```python
from build123d import *

# Parameters (mm, degrees)
SKETCH1_W           = 198.12
SKETCH1_H           = 248.92
SKETCH1_R           = 2.5
BOSS_EXTRUDE1_DEPTH = 3.175
SKETCH2_R           = 6.35
CUT_EXTRUDE1_DEPTH  = 4.175


with BuildPart() as part:
    # Sketch1 → Boss-Extrude1 (new body)
    with BuildSketch(Plane.XY):
        with Locations((0, -152.4)):
            Rectangle(SKETCH1_W, SKETCH1_H)
        with Locations((-76.2, -260.35)):
            Circle(SKETCH1_R, mode=Mode.SUBTRACT)
        with Locations((-76.2, -38.1)):
            Circle(SKETCH1_R, mode=Mode.SUBTRACT)
        with Locations((76.2, -38.1)):
            Circle(SKETCH1_R, mode=Mode.SUBTRACT)
        with Locations((76.2, -260.35)):
            Circle(SKETCH1_R, mode=Mode.SUBTRACT)
    extrude(amount=BOSS_EXTRUDE1_DEPTH)

    # Sketch2 → Cut-Extrude1 (cut, through all)
    with BuildSketch(Plane.XY.offset(3.175)):
        with Locations((-54.61, -78.74)):
            Circle(SKETCH2_R)
        with Locations((54.61, -78.74)):
            Circle(SKETCH2_R)
    extrude(amount=-CUT_EXTRUDE1_DEPTH, mode=Mode.SUBTRACT)


solid = part.part
```
Build history of the part. All positions in model axes, mm. Round coordinates to 2 decimals unless told otherwise and drop trailing zeros. Write each loop counter-clockwise with the first axis right and the second up, starting at its lowest first coordinate (ties: lowest second). Pieces come first, ordered by that corner, then holes.
1) Band-saw the part on A-A, the plane x = -54.61. List the corners of the cut face in (y, z) (3 decimals), and give its area (3 significant figures).
2) Pin check, flat tip, straight feed: pin 1 (3 mm diameter, centred on x = 76.2, y = -260.35, fed in from +Z). Stop position of the tip, or through.
3) Mould opens along X. For faces 1 (the cylindrical face through (-76.53, -35.62, 1.57)), 2 (the flat face through (-1, -151, 3.175)) say: +X half, -X half, draft (parallel to the pull), parting line (faces both ways), or undercut.
4) Drill centre lines: probe 1 along Y at (x, z) = (-76.2, 1.35); probe 2 along X at (y, z) = (-260.35, 2.55); probe 3 along Y at (x, z) = (54.61, 2.05). Where is each one in solid material? Low to high.
5) Band-saw the part on B-B, the plane y = -78.74. List the corners of the cut face in (x, z) (3 decimals).
Ans:
1. outline: (-276.86, 0) - (-85.09, 0) - (-85.09, 3.175) - (-276.86, 3.175) - close; (-72.39, 0) - (-27.94, 0) - (-27.94, 3.175) - (-72.39, 3.175) - close
1. area: 750 mm2
2. pin 1: passes through
3. face 1: undercut
3. face 2: draft
4. probe 1: y = -276.86 to -262.85, -257.85 to -40.6, -35.6 to -27.94
4. probe 2: x = -99.06 to -78.7, -73.7 to 73.7, 78.7 to 99.06
4. probe 3: y = -276.86 to -85.09, -72.39 to -27.94
5. outline: (-99.06, 0) - (-60.96, 0) - (-60.96, 3.175) - (-99.06, 3.175) - close; (-48.26, 0) - (48.26, 0) - (48.26, 3.175) - (-48.26, 3.175) - close; (60.96, 0) - (99.06, 0) - (99.06, 3.175) - (60.96, 3.175) - close
